Could you check a few things on this drawing? It's one solid part, dimensions in mm from its lowest x, y, z. A direction names the side the tool comes from. Give positions to 0.01 mm unless a question says otherwise; leave off trailing zeros. Loops run counter-clockwise (first coordinate to the right, second up) from the corner with the lowest first, then second, coordinate; pieces in that order, holes last. Notation, with made-up numbers: (65, 29) - (69, 29) arc R23 cw to (69, 52) - close; hole circle Ø3 at (33, 48.5). An arc over 180 degrees is marked (long way). Return JSON: item names as keys, results as strings. Group by question number.
(1) If we section it at A-A (z = 4.5): Please give me the cut outline in (x, y).
(2) I need wall thicknesses on probe 1 along X at (y, z) = (44, 32); probe 2 along Y at (x, z) = (44.5, 7); probe 3 along Y at (x, z) = (130, 17). Which ranges of each line are inside material? Lowest first, please. Write a range as [from, to].
(3) If we section it at C-C (z = 32.5): Please give me the cut outline in (x, y) (3 decimals), then the cut area to 3 significant figures.
(4) If we mould it in two halves opening along X, with no side actions, what happens to the marked faces 4, 5 and 6? For each: released by +X, released by -X, zero draft, split by the parting line, or undercut.
(5) For P1, Ø5.5, axis at x = 90, y = 77, coming from the +Z side; P2, Ø4, axis at x = 113, z = 34.5, coming from the -Y side; P3, Ø15, axis at x = 54.5, y = 46.5, coming from the -Z side, each with a flat end and sliding along its axis, tell me the tip position at first contact or that it passes through.
(6) If we section it at D-D (x = 124.5): Please give me the cut outline in (y, z).
(7) On a 3-axis mill with a long thin cutter (end or side, diameter ignored), from which of +Z, -Z, +X, -X, +Y, -Y can I reach the whole of each face in a straight line? I mean the marked faces 1, 2 and 3. Say none if no direction works.
(8) If we section it at B-B (y = 46.5): Please give me the cut outline in (x, z), then the cut area to 3 significant figures.
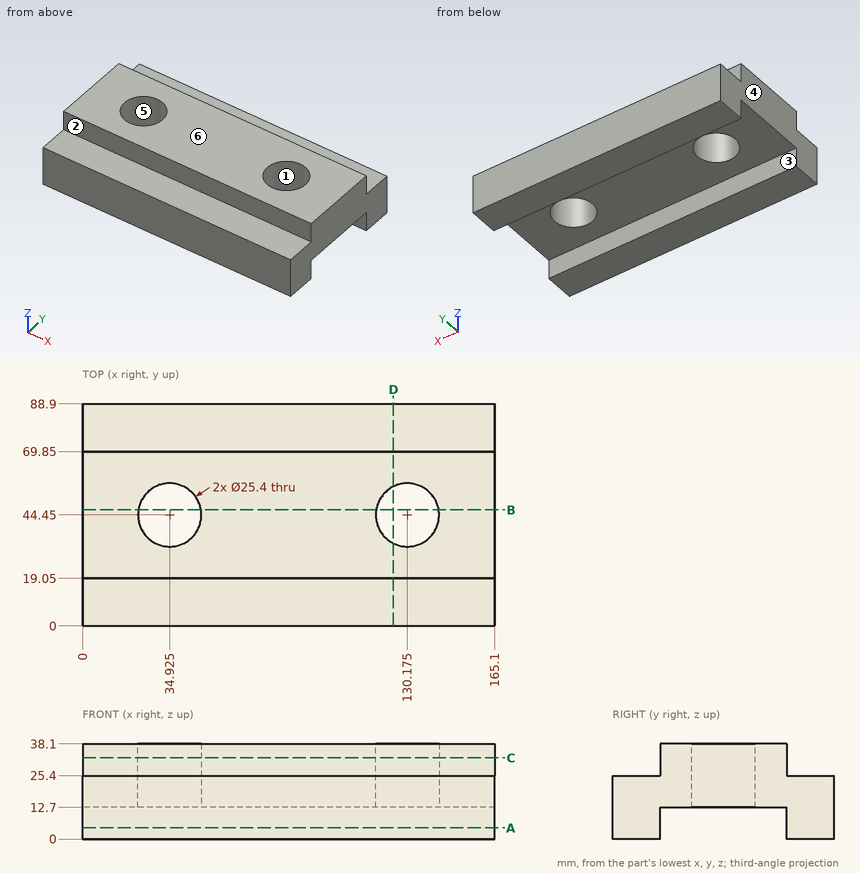
Values:
{
 "1": {"outline": "(0, 0) - (165.1, 0) - (165.1, 19.05) - (0, 19.05) - close; (0, 69.85) - (165.1, 69.85) - (165.1, 88.9) - (0, 88.9) - close"},
 "2": {"probe 1": "[0, 22.23], [47.62, 117.48], [142.87, 165.1]", "probe 2": "[0, 19.05], [69.85, 88.9]", "probe 3": "[0, 31.75], [57.15, 88.9]"},
 "3": {"outline": "(0, 19.05) - (165.1, 19.05) - (165.1, 69.85) - (0, 69.85) - close; hole circle Ø25.4 at (34.925, 44.45); hole circle Ø25.4 at (130.175, 44.45)", "area": "7,370 mm2"},
 "4": {"face 4": "released by -X", "face 5": "undercut", "face 6": "zero draft"},
 "5": {"P1": "z = 25.4", "P2": "y = 19.05", "P3": "z = 12.7"},
 "6": {"outline": "(0, 0) - (19.05, 0) - (19.05, 12.7) - (33.09, 12.7) - (33.09, 38.1) - (19.05, 38.1) - (19.05, 25.4) - (0, 25.4) - close; (55.81, 12.7) - (69.85, 12.7) - (69.85, 0) - (88.9, 0) - (88.9, 25.4) - (69.85, 25.4) - (69.85, 38.1) - (55.81, 38.1) - close"},
 "7": {"face 1": "+Z, -Z", "face 2": "+Z, +X, -X, -Y", "face 3": "-Z, +X, -X"},
 "8": {"outline": "(0, 12.7) - (22.39, 12.7) - (22.39, 38.1) - (0, 38.1) - close; (47.46, 12.7) - (117.64, 12.7) - (117.64, 38.1) - (47.46, 38.1) - close; (142.71, 12.7) - (165.1, 12.7) - (165.1, 38.1) - (142.71, 38.1) - close", "area": "2,920 mm2"}
}
